CAD build for the part. Positions are in the model's coordinates, mm. Face numbers are marked on the shaded views. Give positions to 0.01 mm unless a question says otherwise; leave off trailing zeros. Order: outer loops, then holes, each group sorted by start corner. A loop starts at its lowest first (then second) coordinate and runs counter-clockwise, first axis right, second up. Notation, with made-up numbers: (59, -14) -> (87, -14) arc R30 cw to (87, 25) -> close; hole circle Ø3 at (68, 50.5). An arc over 180 degrees is marked (long way). Answer as CSV lines item,"result".
Autodesk Inventor part; units mm, degrees
ref_plane "Plano de trabajo1" through (0, 0, -40) normal (0, 0, -1) x (-1, 0, 0)
ref_plane "Plano de trabajo2" through (0, 0, -20) normal (0, 0, -1) x (-1, 0, 0)
ref_plane "YZ Plane" through (0, 0, 0) normal (1, 0, 0) x (0, 1, 0)
sketch "Boceto1" plane through (0, 0, 0) normal (0, 0, 1) x (1, 0, 0)
  line L0 (-91, 11.75) -> (-91, -11.75)
  line L1 (-89, -13.75) -> (-33, -13.75)
  line L2 (-31, -11.75) -> (-31, -12)
  line L3 (-29, -10) -> (29, -10)
  line L4 (31, -12) -> (31, -11.75)
  line L5 (33, -13.75) -> (89, -13.75)
  line L6 (91, -11.75) -> (91, 11.75)
  line L7 (89, 13.75) -> (33, 13.75)
  line L8 (31, 11.75) -> (31, 12)
  line L9 (29, 10) -> (-29, 10)
  line L10 (-31, 12) -> (-31, 11.75)
  line L11 (-33, 13.75) -> (-89, 13.75)
  line L12 (0, 0) -> (0, 52.9432) construction
  line L13 (0, 0) -> (-66, 0) construction
  arc A0 (-89, 13.75) -> (-91, 11.75) centre (-89, 11.75) ccw
  arc A1 (-91, -11.75) -> (-89, -13.75) centre (-89, -11.75) ccw
  arc A2 (-33, -13.75) -> (-31, -11.75) centre (-33, -11.75) ccw
  arc A3 (-29, -10) -> (-31, -12) centre (-29, -12) ccw
  arc A4 (-31, 12) -> (-29, 10) centre (-29, 12) ccw
  arc A5 (-31, 11.75) -> (-33, 13.75) centre (-33, 11.75) ccw
  arc A6 (29, 10) -> (31, 12) centre (29, 12) ccw
  arc A7 (33, 13.75) -> (31, 11.75) centre (33, 11.75) ccw
  arc A8 (31, -12) -> (29, -10) centre (29, -12) ccw
  arc A9 (31, -11.75) -> (33, -13.75) centre (33, -11.75) ccw
  arc A10 (89, -13.75) -> (91, -11.75) centre (89, -11.75) ccw
  arc A11 (91, 11.75) -> (89, 13.75) centre (89, 11.75) ccw
  point P0 (-91, 13.75)
  point P1 (-91, -13.75)
  point P2 (-31, -13.75)
  point P3 (91, -13.75)
  point P4 (91, 13.75)
  point P5 (31, 13.75)
  point P6 (31, 10)
  point P7 (-31, 10)
  point P8 (-31, 13.75)
  dimension "d0" = 182
  dimension "d1" = 60
  dimension "d3" = 27.5
  dimension "d4" = 20
  dimension "d5" = 2
  dimension "d6" = 27.5
  dimension "d7" = 2
extrude "Extrusión1" add sketch "Boceto1" along normal blind 3
sketch "Boceto2" plane through (0, 0, 3) normal (0, 0, 1) x (1, 0, 0)
  circle A0 centre (-20, 0) radius 2.5
  circle A1 centre (20, 0) radius 2.5
  line L0 (0, 0) -> (0, 32) construction
  dimension "d10" = 5
  dimension "d11" = 5
  dimension "d12" = 40
extrude "Extrusión2" cut sketch "Boceto2" against normal blind 3
ref_plane "Plano de trabajo1" through (0, 0, -40) normal (0, 0, -1) x (-1, 0, 0)
sketch "Boceto3" plane through (0, 0, -40) normal (0, 0, -1) x (-1, 0, 0)
  line L0 (-86, 1.75) -> (-86, -1.75)
  line L1 (-74, -13.75) -> (-33, -13.75)
  line L2 (-31, -11.75) -> (-31, -12)
  line L3 (-29, -10) -> (29, -10)
  line L4 (31, -12) -> (31, -11.75)
  line L5 (33, -13.75) -> (54, -13.75)
  line L6 (66, -1.75) -> (66, 1.75)
  line L7 (54, 13.75) -> (33, 13.75)
  line L8 (31, 11.75) -> (31, 10)
  line L9 (31, 10) -> (-29, 10)
  line L10 (-31, 12) -> (-31, 11.75)
  line L11 (-33, 13.75) -> (-74, 13.75)
  line L12 (0, 0) -> (0, 26) construction
  line L13 (0, 0) -> (49, 0) construction
  arc A0 (-74, 13.75) -> (-86, 1.75) centre (-74, 1.75) ccw
  arc A1 (-86, -1.75) -> (-74, -13.75) centre (-74, -1.75) ccw
  arc A2 (66, 1.75) -> (54, 13.75) centre (54, 1.75) ccw
  arc A3 (54, -13.75) -> (66, -1.75) centre (54, -1.75) ccw
  arc A4 (-31, 11.75) -> (-33, 13.75) centre (-33, 11.75) ccw
  arc A5 (-31, 12) -> (-29, 10) centre (-29, 12) ccw
  arc A6 (-29, -10) -> (-31, -12) centre (-29, -12) ccw
  arc A7 (-33, -13.75) -> (-31, -11.75) centre (-33, -11.75) ccw
  arc A8 (33, 13.75) -> (31, 11.75) centre (33, 11.75) ccw
  arc A9 (31, -11.75) -> (33, -13.75) centre (33, -11.75) ccw
  arc A10 (31, -12) -> (29, -10) centre (29, -12) ccw
  point P0 (-86, 13.75)
  point P1 (-86, -13.75)
  point P2 (66, -13.75)
  point P3 (66, 13.75)
  point P4 (31, 13.75)
  point P5 (-31, 10)
  point P6 (-31, 13.75)
  dimension "d16" = 27.5
  dimension "d17" = 27.5
  dimension "d18" = 152
  dimension "d19" = 55
  dimension "d21" = 62
  dimension "d22" = 20
  dimension "d23" = 12
  dimension "d24" = 2
extrude "Extrusión3" add sketch "Boceto3" along normal blind 3
sketch "Boceto4" plane through (0, 0, -43) normal (0, 0, -1) x (-1, 0, 0)
  circle A0 centre (-20, 0) radius 2.5
  circle A1 centre (20, 0) radius 2.5
  point P0 (0, 0)
extrude "Extrusión4" cut sketch "Boceto4" against normal blind 3
sketch "Boceto5" plane through (0, 0, 3) normal (0, 0, 1) x (1, 0, 0)
  line L0 (-51, 21) -> (-51, -25) construction
  line L1 (71, 20) -> (71, -24) construction
  line L2 (31, -12) -> (31, -11.75)
  circle A0 centre (-51, 0) radius 2.5
  circle A1 centre (71, 0) radius 2.5
  line L3 (-91, 11.75) -> (-91, -11.75)
  point P0 (31, -11.875)
  dimension "d32" = 40
  dimension "d34" = 5
  dimension "d35" = 5
  dimension "d46" = 40
extrude "Extrusión5" cut sketch "Boceto5" against normal up to surface (46 mm away)
sketch "Boceto6" plane through (0, 0, -43) normal (0, 0, -1) x (-1, 0, 0)
  circle A0 centre (51, 0) radius 2.5
  line L0 (31, 11.75) -> (31, 10)
  point P0 (0, 0)
  point P1 (31, 10.875)
  dimension "d38" = 5
  dimension "d39" = 20
extrude "Extrusión6" cut sketch "Boceto6" against normal blind 3
ref_plane "Plano de trabajo2" through (0, 0, -20) normal (0, 0, -1) x (-1, 0, 0)
sketch "Boceto7" plane through (0, 0, -20) normal (0, 0, -1) x (-1, 0, 0)
  circle A0 centre (20, 0) radius 2.5
  circle A1 centre (-20, 0) radius 2.5
  point P0 (0, 0)
extrude "Extrusión7" add sketch "Boceto7" along normal mid plane 46
sketch "Boceto8" plane through (0, 0, 3) normal (0, 0, 1) x (1, 0, 0)
  line L0 (38.7008, -6.0818) -> (38.7008, 17.3731) construction
  line L1 (38.7008, 17.3731) -> (57.2312, 17.3731) construction
  line L2 (57.2312, 17.3731) -> (57.2312, -6.0818) construction
  line L3 (57.2312, -6.0818) -> (38.7008, -6.0818) construction
  line L4 (46.5776, 2.5146) -> (46.5776, 1.0851)
  line L5 (46.5776, 1.0851) -> (50.7008, 1.0851)
  line L6 (50.7008, 1.0851) -> (50.7008, -0.461)
  line L7 (50.7008, -0.461) -> (46.5776, -0.461)
  line L8 (46.5776, -0.461) -> (46.5776, -5.7609)
  line L9 (46.5776, -5.7609) -> (44.8855, -5.7609)
  line L10 (44.8855, -5.7609) -> (38.7008, -0.393)
  line L11 (38.7008, -0.393) -> (38.7008, 1.0851)
  line L12 (38.7008, 1.0851) -> (45.2842, 1.0851)
  line L13 (45.2842, 1.0851) -> (45.2842, 2.5146)
  line L14 (45.2842, 2.5146) -> (46.5776, 2.5146)
  line L15 (45.2842, -0.461) -> (40.597, -0.461)
  line L16 (40.597, -0.461) -> (45.2842, -4.4967)
  line L17 (45.2842, -4.4967) -> (45.2842, -0.461)
  point P0 (0, 0)
extrude "Extrusión8" cut sketch "Boceto8" against normal blind 0.5
sketch "Boceto9" plane through (0, 0, 3) normal (0, 0, 1) x (1, 0, 0)
  line L0 (-83, 10.6047) -> (-42.6, 10.6047)
  line L1 (-42.6, 10.6047) -> (-42.6, -9.3953)
  line L2 (-42.6, -9.3953) -> (-83, -9.3953)
  line L3 (-83, -9.3953) -> (-83, 10.6047)
  line L4 (-91, 11.75) -> (-91, -11.75) construction
  point P0 (0, 0)
  dimension "d47" = 40.4
  dimension "d48" = 20
  dimension "d49" = 8
extrude "Extrusión9" cut sketch "Boceto9" against normal up to surface (3 mm away)
sketch "Boceto10" plane through (0, 0, -43) normal (0, 0, -1) x (-1, 0, 0)
  line L0 (-79.4, 10) -> (-39, 10)
  line L1 (-39, 10) -> (-39, -10)
  line L2 (-39, -10) -> (-79.4, -10)
  line L3 (-79.4, -10) -> (-79.4, 10)
  line L4 (-71, 0) -> (-43, 0) construction
  line L5 (-31, 12) -> (-31, 11.75)
  point P0 (0, 0)
  point P1 (-31, 11.875)
  dimension "d52" = 40.4
  dimension "d53" = 20
  dimension "d54" = 8
extrude "Extrusión10" cut sketch "Boceto10" against normal blind 3
equation "\"Radio_pliegue\" = Grosor"
equation "\"Anchura_desahogo_plegado\" = Grosor"
equation "\"Profundidad_desahogo_plegado\" = 0.5 * Grosor"
equation "\"Tamaño_destalonado\" = 4 * Grosor"
equation "\"Remanente_mínimo\" = 2 * Grosor"
equation "\"Radiodetransición\" = Radio_pliegue"
equation "\"Tamaño_de_radio_de_Jacobi\" = Radio_pliegue"
equation "\"TamañoSeparación\" = Grosor"
properties part number "Pieza_eslabon_4"
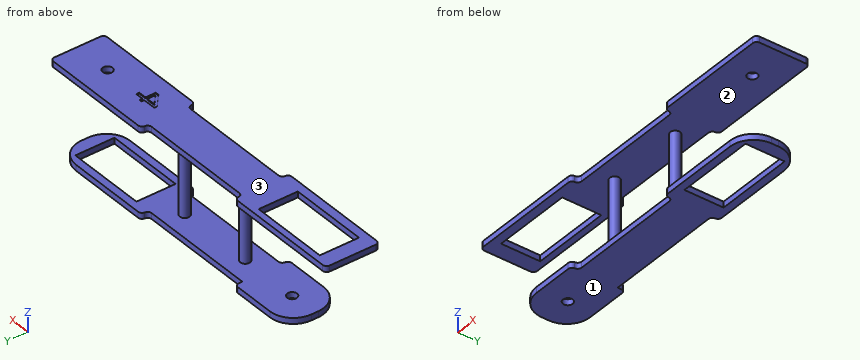
1) Pin check, flat tips, straight feed: P1, Ø1.5, axis at x = -3.5, z = 2, coming from the +Y side; P2, Ø4, axis at y = -1.5, z = -24.5, coming from the +X side; P3, Ø3.5, axis at x = 0, z = 2, coming from the -Y side. Stop position of each tip, or through.
Data:
P1,"stops at y = 10"
P2,"stops at x = 22.5"
P3,"stops at y = -10"
2) Band-saw the part on A-A, the plane x = -51. Write the cut outline in (y, z), then the cut area to 3 significant figures.
Data:
outline,"(-13.75, -43) -> (-2.5, -43) -> (-2.5, -40) -> (-13.75, -40) -> close; (-13.75, 0) -> (-9.4, 0) -> (-9.4, 3) -> (-13.75, 3) -> close; (2.5, -43) -> (13.75, -43) -> (13.75, -40) -> (2.5, -40) -> close; (10.6, 0) -> (13.75, 0) -> (13.75, 3) -> (10.6, 3) -> close"
area,"90.0 mm2"
3) Pull direction Z, two halves, no side cores. Call the marked faces 1, 2 and 3: pulls with the +Z half, pulls with the -Z half, needs draft (parallel to the pull), parting line crosses it, or undercut.
Data:
face 1,"pulls with the -Z half"
face 2,"undercut"
face 3,"pulls with the +Z half"
4) Wall check: line 1 along X through (y, z) = (0, -41.05); line 2 along Z through (x, y) = (-22, 5); line 3 along Y through (x, z) = (71, 1.7). Give the ranges that are in metal, low to high. Write a range as [from, to].
Data:
line 1,"x = [-66, -53.5], [-48.5, 39], [79.4, 86]"
line 2,"z = [-43, -40], [0, 3]"
line 3,"y = [-13.75, -2.5], [2.5, 13.75]"
5) Band-saw the part on D-D, the plane x = -20. Write the cut outline in (y, z), then the cut area to 3 significant figures.
Data:
outline,"(-10, -43) -> (10, -43) -> (10, -40) -> (2.5, -40) -> (2.5, 0) -> (10, 0) -> (10, 3) -> (-10, 3) -> (-10, 0) -> (-2.5, 0) -> (-2.5, -40) -> (-10, -40) -> close"
area,"320 mm2"
6) Band-saw the part on C-C, the plane z = -37. Write the cut outline in (x, y).
Data:
outline,"circle Ø5 at (-20, 0); circle Ø5 at (20, 0)"
7) Band-saw the part on B-B, the plane x = 57. Write the cut outline in (y, z), then the cut area to 3 significant figures.
Data:
outline,"(-13.75, -43) -> (-10, -43) -> (-10, -40) -> (-13.75, -40) -> close; (-13.75, 0) -> (13.75, 0) -> (13.75, 3) -> (-13.75, 3) -> close; (10, -43) -> (13.75, -43) -> (13.75, -40) -> (10, -40) -> close"
area,"105 mm2"
